Design review of the part built by this model. Coordinates are the model's own, in mm. A direction names the side the tool comes from. Coordinates: 2 decimals unless noted, no trailing zeros. Loops run counter-clockwise (first coordinate to the right, second up) from the corner with the lowest first, then second, coordinate; pieces in that order, holes last. Notation, with made-up numbers: M 59.5,-30 L 81.5,-30 A22 cw 81.5,-18 Z; hole C 38.5,74.5 d10. An arc over 180 degrees is marked long. Put each result on its own line as item: value. Start each with the question number.
(1) For probe 1 along Z at (x, y) = (0, 43.05); probe 2 along Z at (x, y) = (0, 44.8); probe 3 along X at (y, z) = (44.3, 22), list the stretches that pass through material, from the lowest coordinate up. Write a range as [from, to].
(2) Take a section at B-B, the plane x = 28.5. Give the boundary of the cut face in (y, z).
(3) Clearance check with flat-ended pins moving along their axes: pin 1 (2 mm diameter, centred on x = 1, z = 27, fed in from -Y); pin 2 (7 mm diameter, centred on x = -6.5, z = 24, fed in from +Y); pin 3 (1 mm diameter, centred on y = 46.5, z = 9, fed in from -X); pin 4 (1 mm diameter, centred on x = -31.5, y = 44.5, fed in from +Z). State where each tip first meets the part, or that it passes through.
(4) Take a section at A-A, the plane z = 12.5. Give the boundary of the cut face in (x, y).
(5) The part is to be moulded in two halves that separate along Z. For faces 6 (the flat face through (51.479, 45.672, 20.576)), 7 (the flat face through (-52.905, 45.672, 13.441)), 8 (the cylindrical face through (-17.31, 45.73, 30.43)), 9 (the cylindrical face through (-8.098, 45.728, 19.486)), say which applies: +Z half, -Z half, draft (parallel to the pull), parting line (faces both ways), or undercut.
(6) For faces 1 (the cylindrical face through (49.215, 45.728, 24.381)), 2 (the flat face through (-55, 46, -17)), 3 (the flat face through (-4.05, 45.5, 24.66)), 4 (the flat face through (0, 47.7, 19)), 5 (the flat face through (-50.94, 45.73, -4.67)), list the 3-axis set-ups (+Z, -Z, +X, -X, +Y, -Y) from which the entire face can be reached by the end or side of a thin tool; tool diameter is ignored.
```python
from build123d import *

# Parameters (mm, degrees)
PAD071_DEPTH       = 4
PAD069_DEPTH       = 4
POCKET003051_DEPTH = 2.2
PAD070_DEPTH       = 4
SKETCH116_R        = 3.9
POCKET003052_DEPTH = 10
SKETCH118_R        = 5.5
SKETCH118_R_2      = 3.891802
PAD072_DEPTH       = 1
SKETCH119_W        = 122.5
SKETCH119_H        = 2
POCKET003053_DEPTH = 5


with BuildPart() as central_leg_insect_add001:
    # Sketch117 → Pad071 (new body)
    with BuildSketch(Plane.XZ.offset(-43.7)):
        Polygon((-58.503296, -18.004301), (-53.997036, -18.004301), (-48.744877, 15.965196), (-44.5658, 27.943165), (-41.53833, 30.02603), (-31.626242, 31.40176), (-21.017805, 29.65671), (-18.990362, 30.401161), (-27.13097, 35.111233), (-22.936073, 30.916338), (-29.003351, 32.984856), (-36.116627, 34.99157), (-32.000511, 32.969288), (-34.972557, 32.969288), (-41.352551, 34.221657), (-37, 32.591213), (-43, 31.631081), (-48.636986, 29.73181), (-44, 30.22826), (-46, 29.721722), (-51, 25.793291), (-47.464714, 26.759798), (-49.314915, 23.492535), (-53.390827, 18), (-50, 21), (-51, 16.646269), (-54.355499, 11), (-51.685394, 14), (-52.498241, 9), (-55.106018, 4.606695), (-52.495518, 7), (-53.502594, 2), (-56, -2.398534), (-53.492668, 0), (-54.22747, -6), (-56.500393, -9.69598), (-54.497387, -8), (-55, -14), (-58.503296, -17.601286), align=None)
    extrude(amount=-PAD071_DEPTH)


with BuildPart() as quarter_central_leg_servo_support001:
    # Sketch113 → Pad069 (new body)
    with BuildSketch(Plane(origin=(0, 47.7, 24.6), x_dir=(-1, 0, 0), z_dir=(0, 1, 0))):
        with BuildLine():
            ThreePointArc((15.732627, 3), (7.987175, 5.135172), (0, 6.004658))
            Line((0, 6.004658), (0, 4.275313))
            Line((0, 4.275313), (0, 0))
            Line((16.774147, 0), (0, 0))
            Line((18.088162, 0), (16.774147, 0))
            ThreePointArc((18.088162, 0), (17.428911, 1.907128), (15.732627, 3))
        make_face()
    extrude(amount=-PAD069_DEPTH)

    # Sketch114 → Pocket003051 (cut)
    with BuildSketch(Plane(origin=(0, 47.7, 24.6), x_dir=(-1, 0, 0), z_dir=(0, 1, 0))):
        with BuildLine():
            Line((0, 4.49111), (15.744728, 2.000001))
            ThreePointArc((17.134156, 0), (16.75271, 1.217632), (15.744728, 2.000001))
            Line((17.134156, 0), (0, 0))
            Line((0, 0), (0, 4.49111))
        make_face()
    extrude(amount=-POCKET003051_DEPTH, mode=Mode.SUBTRACT)


with BuildPart() as half_leg_insect001:
    # Part__Mirroring009: instance of quarter_central_leg_servo_support001
    add(quarter_central_leg_servo_support001.part.mirror(Plane(origin=(0, 0, 24.6), x_dir=(0, 1, 0), z_dir=(0, 0, 1))))

    # Fusion007042: union quarter_central_leg_servo_support001
    add(quarter_central_leg_servo_support001.part)

    # Sketch115 → Pad070 (new body)
    with BuildSketch(Plane(origin=(0, 47.7, 0), x_dir=(-1, 0, 0), z_dir=(0, 1, 0))):
        with BuildLine():
            Line((52.452988, -18.000002), (58.497849, -18.000002))
            Line((58.497849, -18.000002), (58.497849, -17.584217))
            ThreePointArc((54.988709, -14), (56.535613, -15.995425), (58.497849, -17.584217))
            Line((54.988709, -14), (52.759255, 8.35829))
            ThreePointArc((52.759255, 8.35829), (51.202034, 17.133916), (48.77817, 25.710712))
            ThreePointArc((48.77817, 25.710712), (46.1643, 29.690829), (42.000002, 32))
            ThreePointArc((42.000002, 32), (27.145674, 33.002324), (13.00001, 28.359486))
            Line((16, 27.29138), (13.00001, 28.359486))
            ThreePointArc((41.999998, 28.999997), (28.860359, 30.270585), (16, 27.29138))
            ThreePointArc((44.999996, 25.769916), (43.714535, 27.584213), (41.999998, 28.999997))
            ThreePointArc((49.501895, 8.000017), (47.87481, 17.043019), (44.999996, 25.769916))
            Line((52.452988, -18.000002), (49.501895, 8.000017))
        make_face()
    extrude(amount=-PAD070_DEPTH)

    # Fusion007043: union central_leg_insect_add001
    add(central_leg_insect_add001.part)


with BuildPart() as obj1:
    # Part__Mirroring010: instance of half_leg_insect001
    add(half_leg_insect001.part.mirror(Plane(origin=(0, 0, 0), x_dir=(0, -1, 0), z_dir=(1, 0, 0))))

    # Fusion007044: union half_leg_insect001
    add(half_leg_insect001.part)

    # Sketch116 → Pocket003052 (cut)
    with BuildSketch(Plane(origin=(0, 45.5, 0), x_dir=(-1, 0, 0), z_dir=(0, 1, 0))):
        with Locations((0, 24.473736)):
            Circle(SKETCH116_R)
    extrude(amount=-POCKET003052_DEPTH, mode=Mode.SUBTRACT)

    # Sketch118 → Pad072 (new body)
    with BuildSketch(Plane.XZ.offset(-43.7)):
        with Locations((0, 24.5)):
            Circle(SKETCH118_R)
        with Locations((0, 24.5)):
            Circle(SKETCH118_R_2, mode=Mode.SUBTRACT)
    extrude(amount=PAD072_DEPTH)

    # Sketch119 → Pocket003053 (cut)
    with BuildSketch(Plane(origin=(0, 47.7, 0), x_dir=(-1, 0, 0), z_dir=(0, 1, 0))):
        with Locations((1.75, -18)):
            Rectangle(SKETCH119_W, SKETCH119_H)
    extrude(amount=-POCKET003053_DEPTH, mode=Mode.SUBTRACT)


solid = obj1.part
```
Computed values:
1. probe 1: z = [19, 20.61], [28.39, 30]
1. probe 2: z = [18.6, 20.57], [28.37, 30.6]
1. probe 3: x = [-50.42, -46.41], [-16.67, -3.02], [3.02, 16.67], [46.41, 50.42]
2. outline: M 43.7,30.25 L 47.7,30.25 L 47.7,33.15 L 43.7,33.15 Z
3. pin 1: passes through
3. pin 2: stops at y = 47.7
3. pin 3: stops at x = -52.8
3. pin 4: stops at z = 33.83
4. outline: M -53.46,43.7 L -53.02,43.7 L -53.02,47.7 L -53.46,47.7 Z; M -52.14,43.7 L -48.86,43.7 L -48.86,47.7 L -52.14,47.7 Z; M 48.86,43.7 L 52.14,43.7 L 52.14,47.7 L 48.86,47.7 Z; M 53.02,43.7 L 53.46,43.7 L 53.46,47.7 L 53.02,47.7 Z
5. face 6: undercut
5. face 7: undercut
5. face 8: +Z half
5. face 9: -Z half
6. face 1: +X, +Y, -Y
6. face 2: -Z, +X, -X, +Y, -Y
6. face 3: +Y
6. face 4: +Z, -Z, +X, -X, +Y
6. face 5: -Z, +Y, -Y
